Can you work these out from the model? Positions are in its coordinate system, mm. Face numbers are marked on the shaded views. A direction names the side the tool comes from. Round coordinates to 2 decimals unless told otherwise and drop trailing zeros. Order: outer loops, then holes, each group sorted by start corner. A loop starts at its lowest first (then second) coordinate and runs counter-clockwise, first axis right, second up. Notation, with made-up numbers: M 74,87 L 91,87 A18 ccw 91,109 Z; hole C -28,7.25 d6. An arc over 180 degrees is marked long. Answer as a JSON object with one key per item and string values. Group by question number.
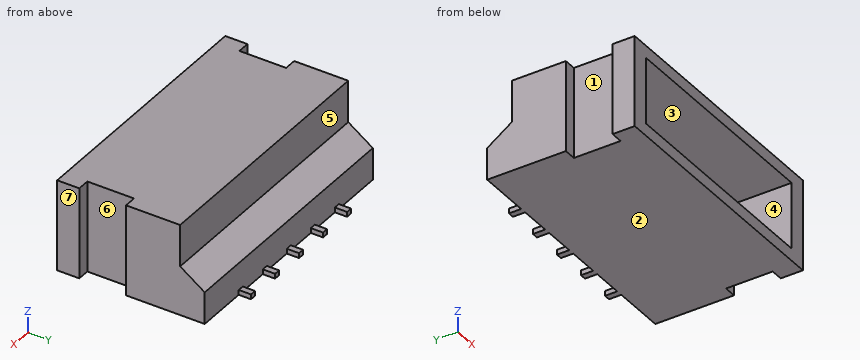
from build123d import *

# Parameters (mm, degrees)
SKETCH_W            = 10.5
SKETCH_H            = 6
PAD_DEPTH           = 3.7
SKETCH001_W         = 0.25
SKETCH001_H         = 0.5
PAD001_DEPTH        = 0.2
LINEARPATTERN_COUNT = 5
LINEARPATTERN_PITCH = 1.5
POCKET_DEPTH        = 5.251
POCKET_DEPTH_BACK   = -5.251
SKETCH003_W         = 0.5
SKETCH003_H         = 1.9
POCKET001_DEPTH     = 29.48394
SKETCH004_W         = 9.1
SKETCH004_H         = 2.7
POCKET002_DEPTH     = 4


with BuildPart() as part:
    # Sketch → Pad (new body)
    with BuildSketch(Plane.XY):
        with Locations((0, -0.9)):
            Rectangle(SKETCH_W, SKETCH_H)
    extrude(amount=PAD_DEPTH)

    # Sketch001 → Pad001 (join)
    with BuildSketch(Plane.XY):
        with Locations((-3, 2.35)):
            Rectangle(SKETCH001_W, SKETCH001_H)
    pad001 = extrude(amount=PAD001_DEPTH)

    # LinearPattern: Pad001 ×5
    with Locations(*[(i * LINEARPATTERN_PITCH, 0, 0) for i in range(1, LINEARPATTERN_COUNT)]):
        add(pad001)

    # Sketch002 → Pocket (cut, two sides)
    with BuildSketch(Plane.YZ) as pocket_sk:
        Polygon((1.1, 3.7), (2.1, 3.7), (2.1, 1.3), (1.1, 2), align=None)
    extrude(amount=-POCKET_DEPTH, mode=Mode.SUBTRACT)
    extrude(pocket_sk.sketch, amount=-POCKET_DEPTH_BACK, mode=Mode.SUBTRACT)

    # Sketch003 → Pocket001 (cut, through all)
    with BuildSketch(Plane.XY):
        with Locations((-5, -2.05)):
            Rectangle(SKETCH003_W, SKETCH003_H)
    pocket001 = extrude(amount=POCKET001_DEPTH, mode=Mode.SUBTRACT)

    # Mirrored: Pocket001 across YZ
    add(pocket001.mirror(Plane.YZ), mode=Mode.SUBTRACT)

    # Sketch004 (on Face18 of Mirrored) → Pocket002 (cut)
    with BuildSketch(Plane.XZ.offset(3.9)):
        with Locations((0, 1.85)):
            Rectangle(SKETCH004_W, SKETCH004_H)
    extrude(amount=-POCKET002_DEPTH, mode=Mode.SUBTRACT)


solid = part.part
Item 1: Suppose I cut it at C-C, the plane z = 2.75. Write out the boundary of the cut face in (x, y), and give its area (3 significant figures).
Item 2: Suppose I cut it at D-D, the plane y = 1.25. Write out the boundary of the cut face in (x, z) (3 decimals), and give its area (3 significant figures).
Item 3: Suppose I cut it at A-A, the plane y = -0.75. Write out the boundary of the cut face in (x, z), and give its area (3 significant figures).
Item 4: On a 3-axis mill with a long thin cutter (end or side, diameter ignored), from which of +Z, -Z, +X, -X, +Y, -Y can I reach the whole of each face in a straight line? I mean the marked faces 5, 6 and 7. Say none if no direction works.
Item 5: I need wall thicknesses on line 1 (X direction, y = 0, z = 2.6); line 2 (Z direction, x = -4.5, y = -2.5); line 3 (X direction, y = -2.25, z = 1.4). Which ranges of each line are inside material? Lowest first, please.
Item 6: If we mould it in two halves opening along X, with no side actions, what happens to the marked faces 1, 2, 3 and 4? For each: +X half, -X half, draft (parallel to the pull), parting line (faces both ways), or undercut.
Item 7: I'm going to push a flat-ended pin straight in: pin 1 Ø0.6 at (y, z) = (-2.5, 2) entering from -X. Where does the tip first touch, or does it pass through?
Item 8: Suppose I cut it at B-B, the plane x = 1.5. Write out the boundary of the cut face in (y, z).
Computed:
{
 "1": {"outline": "M -5.25,-3.9 L -4.55,-3.9 L -4.55,0.1 L 4.55,0.1 L 4.55,-3.9 L 5.25,-3.9 L 5.25,-3 L 4.75,-3 L 4.75,-1.1 L 5.25,-1.1 L 5.25,1.1 L -5.25,1.1 L -5.25,-1.1 L -4.75,-1.1 L -4.75,-3 L -5.25,-3 Z", "area": "14.2 mm^2"},
 "2": {"outline": "M -5.25,0 L 5.25,0 L 5.25,1.895 L -5.25,1.895 Z", "area": "19.9 mm^2"},
 "3": {"outline": "M -5.25,0 L 5.25,0 L 5.25,3.7 L -5.25,3.7 Z; hole M -4.55,0.5 L 4.55,0.5 L 4.55,3.2 L -4.55,3.2 Z", "area": "14.3 mm^2"},
 "4": {"face 5": "+Z, +X, -X, +Y", "face 6": "+Z, -Z, +X", "face 7": "+Z, -Z, +X, +Y, -Y"},
 "5": {"line 1": "x = -5.25 to -4.55, 4.55 to 5.25", "line 2": "z = 0 to 0.5, 3.2 to 3.7", "line 3": "x = -4.75 to -4.55, 4.55 to 4.75"},
 "6": {"face 1": "-X half", "face 2": "draft", "face 3": "undercut", "face 4": "undercut"},
 "7": {"pin 1": "stops at x = -4.75"},
 "8": {"outline": "M -3.9,0 L 2.6,0 L 2.6,0.2 L 2.1,0.2 L 2.1,1.3 L 1.1,2 L 1.1,3.7 L -3.9,3.7 L -3.9,3.2 L 0.1,3.2 L 0.1,0.5 L -3.9,0.5 Z"}
}
